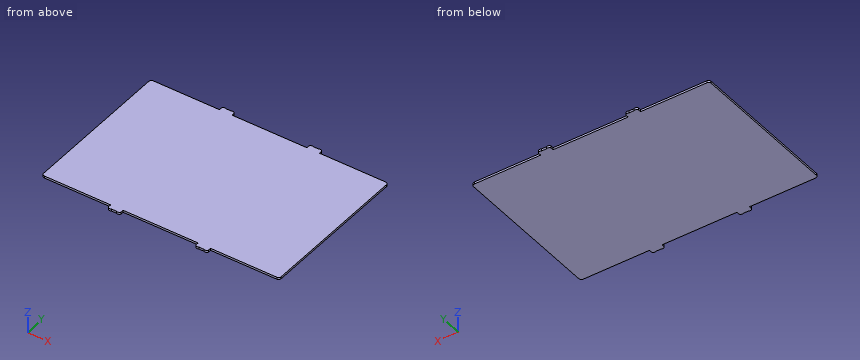
from build123d import *

# Parameters (mm, degrees)
EXTRUDE_1_DEPTH = 4


with BuildPart() as part:
    # Эскиз1 → Бобышка-Вытянуть1 (new body)
    with BuildSketch(Plane.XY):
        with BuildLine():
            Line((177, -66.286621906), (323, -66.286621906))
            Line((323, -66.286621906), (323, -60.286621906))
            ThreePointArc((323, -60.286621906), (326.085786438, -57.836874437), (330, -58.286621906))
            Line((330, -58.286621906), (340, -58.286621906))
            ThreePointArc((340, -58.286621906), (343.914213562, -57.836874437), (347, -60.286621906))
            Line((347, -60.286621906), (347, -66.286621906))
            Line((347, -66.286621906), (476, -66.286621906))
            ThreePointArc((476, -66.286621906), (479.535533906, -67.751088), (481, -71.286621906))
            Line((481, -71.286621906), (481, -361.286621906))
            ThreePointArc((481, -361.286621906), (479.535533906, -364.822155812), (476, -366.286621906))
            Line((476, -366.286621906), (347, -366.286621906))
            Line((347, -366.286621906), (347, -372.286621906))
            ThreePointArc((347, -372.286621906), (343.914213562, -374.736369374), (340, -374.286621906))
            Line((340, -374.286621906), (330, -374.286621906))
            ThreePointArc((330, -374.286621906), (326.085786438, -374.736369374), (323, -372.286621906))
            Line((323, -372.286621906), (323, -366.286621906))
            Line((323, -366.286621906), (177, -366.286621906))
            Line((177, -366.286621906), (177, -372.286621906))
            ThreePointArc((177, -372.286621906), (173.914213562, -374.736369374), (170, -374.286621906))
            Line((170, -374.286621906), (160, -374.286621906))
            ThreePointArc((160, -374.286621906), (156.085786438, -374.736369374), (153, -372.286621906))
            Line((153, -372.286621906), (153, -366.286621906))
            Line((153, -366.286621906), (24, -366.286621906))
            ThreePointArc((24, -366.286621906), (20.464466094, -364.822155812), (19, -361.286621906))
            Line((19, -361.286621906), (19, -71.286621906))
            ThreePointArc((19, -71.286621906), (20.464466094, -67.751088), (24, -66.286621906))
            Line((24, -66.286621906), (153, -66.286621906))
            Line((153, -66.286621906), (153, -60.286621906))
            ThreePointArc((153, -60.286621906), (156.085786438, -57.836874437), (160, -58.286621906))
            Line((160, -58.286621906), (170, -58.286621906))
            ThreePointArc((170, -58.286621906), (173.914213562, -57.836874437), (177, -60.286621906))
            Line((177, -60.286621906), (177, -66.286621906))
        make_face()
    extrude(amount=EXTRUDE_1_DEPTH)


solid = part.part
Input: part model. Units: mm. Frame: model coordinates. Coordinates: 2 decimals unless noted, no trailing zeros. Order: outer loops, then holes, each group sorted by start corner. A loop starts at its lowest first (then second) coordinate and runs counter-clockwise, first axis right, second up. Notation, with made-up numbers: M 17.25,31.5 L 53.25,31.5 A6 ccw 53.25,40.5 Z; hole C -27.5,16 d10. An arc over 180 degrees is marked long. One line per question, with ' | ' between items.
Item 1: Pin query (flat end, axial travel): pin 1 (1.2 mm diameter, centred on x = 285, z = 2, fed in from +Y); pin 2 (1.2 mm diameter, centred on x = 440.5, z = 2, fed in from -Y); pin 3 (2 mm diameter, centred on y = -64.5, z = 1.5, fed in from -X). Return the tip coordinate at first contact, or that it passes through.
Geometry results:
pin 1: stops at y = -66.29 | pin 2: stops at y = -366.29 | pin 3: stops at x = 153
Item 2: Ray query, line 1 along X through (y, z) = (-361.5, 3.3); line 2 along Y through (x, z) = (172, 1.4); line 3 along Y through (x, z) = (230, 3.5). Return the intervals inside material, ascending.
Geometry results:
line 1: x = 19 to 481 | line 2: y = -374.91 to -57.66 | line 3: y = -366.29 to -66.29
Item 3: Section B-B (x = 107.5). Output: boundary loops of the cut face in (y, z), then the cut area to 3 significant figures.
Geometry results:
outline: M -366.29,0 L -66.29,0 L -66.29,4 L -366.29,4 Z | area: 1,200 mm^2
